Input: part model. Units: mm. Frame: model coordinates. A direction names the side the tool comes from. Give positions to 0.01 mm unless a question says otherwise; leave off trailing zeros. Loops run counter-clockwise (first coordinate to the right, second up) from the corner with the lowest first, then second, coordinate; pieces in that order, holes last. Notation, with made-up numbers: M -10.75,85.5 L 21.25,85.5 A13 cw 21.25,102.5 Z; hole C -37,34 d6. An arc over 180 degrees is marked long. Use a Markdown table: item, result. Add a question column.
from build123d import *

# Parameters (mm, degrees)
F0_R     = 4.25
F0_R_2   = 2.25
F1_DEPTH = 8
F0_W     = 15
F0_H     = 2
F2_DEPTH = 21
F3_R     = 2.5
F4_DEPTH = 29.101
F5_R     = 5
F6_R     = 4.25
F7_DEPTH = 4


# Not quite as in the source:
# - a feature names something its author has since deleted; it is built from what else it names


with BuildPart() as f1:
    # F0 (on Top) → F1 (new body)
    with BuildSketch(Plane.XY):
        Polygon((55, -12.55), (70, -12.55), (70, 12.55), (55, 12.55), (-55, 12.55), (-70, 12.55), (-70, -12.55), (-55, -12.55), align=None)
        with Locations((-35, 0)):
            Circle(F0_R, mode=Mode.SUBTRACT)
        with Locations((35, 0)):
            Circle(F0_R, mode=Mode.SUBTRACT)
        with Locations((-35, 0)):
            Circle(F0_R)
        with Locations((-35, 0)):
            Circle(F0_R_2, mode=Mode.SUBTRACT)
        with Locations((35, 0)):
            Circle(F0_R)
        with Locations((35, 0)):
            Circle(F0_R_2, mode=Mode.SUBTRACT)
    extrude(amount=F1_DEPTH)

    # F0 (on Top) → F2 (join)
    with BuildSketch(Plane.XY):
        with Locations((-62.5, -13.55)):
            Rectangle(F0_W, F0_H)
        with Locations((62.5, -13.55)):
            Rectangle(F0_W, F0_H)
        with Locations((-62.5, 13.55)):
            Rectangle(F0_W, F0_H)
        with Locations((62.5, 13.55)):
            Rectangle(F0_W, F0_H)
    extrude(amount=F2_DEPTH)

    # F3 (on face) → F4 (cut, through all)
    with BuildSketch(Plane.XZ.offset(14.55)):
        with Locations((-62, 15)):
            Circle(F3_R)
        with Locations((62, 15)):
            Circle(F3_R)
    extrude(amount=-F4_DEPTH, mode=Mode.SUBTRACT)

    # F5
    f5_edges = [f1.edges().sort_by_distance(p)[0] for p in [
        (-55, -13.55, 21),
        (55, -13.55, 21),
        (-55, 13.55, 21),
        (55, 13.55, 21),
    ]]
    fillet(f5_edges, radius=F5_R)

    # F6 (on face) → F7 (cut)
    with BuildSketch(Plane.XY.offset(8)):
        with Locations((-35, 0)):
            Circle(F6_R)
        with Locations((35, 0)):
            Circle(F6_R)
    extrude(amount=-F7_DEPTH, mode=Mode.SUBTRACT)


solid = f1.part
1) Section query C-C, the plane x = 62. Return the cut outline in (y, z).
2) Reachability of faces 4 (the cylindrical face through (56, 14, 19)), 5 (the flat face through (-64, 12.55, 13)), 6 (the flat face through (1, 12.55, 4)), 7 (the cylindrical face through (-39.246, 0.187, 6.028)) from +Z, -Z, +X, -X, +Y, -Y: full face, straight path, thin tool, end or side. Return the list, or none.
3) Section query A-A, the plane x = 35. Return the cut outline in (y, z), and give its area (3 significant figures).
4) Section query D-D, the plane y = -9. Return the cut outline in (x, z), and give its area (3 significant figures).
5) Contact query for flat-ended pins moving along their axis: P1, Ø1, axis at x = 38.5, y = 10, coming from the +Z side; P2, Ø4, axis at x = 35, y = -1.5, coming from the +Z side; P3, Ø4, axis at x = -1.5, z = 8, coming from the -Y side. Output: stop coordinate, or through.
6) Ray query, line 1 (X direction, y = -12.75, z = 6.75); line 2 (Y direction, x = -35, z = 6.6); line 3 (Z direction, x = 62, y = 13.6). Return the intervals inside material, ascending. Write a range as [from, to].
7) Pull-direction query (X, two-part tool) for faces 1 (the cylindrical face through (-59.69, 13.54, 14.04)), 2 (the flat face through (-63, -14.55, 10)), 3 (the flat face through (70, 0, 6)); classes: pulls with the +X half, pulls with the -X half, needs draft (parallel to the pull), parting line crosses it, or undercut.
8) Section query B-B, the plane y = 0. Return the cut outline in (x, z), and give its area (3 significant figures).
Entries:
| question | item | result |
|---|---|---|
| 1 | outline | M -14.55,0 L 14.55,0 L 14.55,12.5 L 12.55,12.5 L 12.55,8 L -12.55,8 L -12.55,12.5 L -14.55,12.5 Z; M -14.55,17.5 L -12.55,17.5 L -12.55,21 L -14.55,21 Z; M 12.55,17.5 L 14.55,17.5 L 14.55,21 L 12.55,21 Z |
| 2 | face 4 | +Z, +Y, -Y |
| 2 | face 5 | +Z, +X, -X |
| 2 | face 6 | +Z, -Z, +Y |
| 2 | face 7 | +Z |
| 3 | outline | M -12.55,0 L -2.25,0 L -2.25,4 L -4.25,4 L -4.25,8 L -12.55,8 Z; M 2.25,0 L 12.55,0 L 12.55,8 L 4.25,8 L 4.25,4 L 2.25,4 Z |
| 3 | area | 149 mm² |
| 4 | outline | M -70,0 L 70,0 L 70,8 L -70,8 Z |
| 4 | area | 1,120 mm² |
| 5 | P1 | stops at z = 8 |
| 5 | P2 | stops at z = 4 |
| 5 | P3 | stops at y = -12.55 |
| 6 | line 1 | x = [-70, -55], [55, 70] |
| 6 | line 2 | y = [-12.55, -4.25], [4.25, 12.55] |
| 6 | line 3 | z = [0, 12.5], [17.5, 21] |
| 7 | face 1 | undercut |
| 7 | face 2 | needs draft |
| 7 | face 3 | pulls with the +X half |
| 8 | outline | M -70,0 L -37.25,0 L -37.25,4 L -39.25,4 L -39.25,8 L -70,8 Z; M -32.75,0 L 32.75,0 L 32.75,4 L 30.75,4 L 30.75,8 L -30.75,8 L -30.75,4 L -32.75,4 Z; M 37.25,0 L 70,0 L 70,8 L 39.25,8 L 39.25,4 L 37.25,4 Z |
| 8 | area | 1,020 mm² |
